Input: part model. Units: mm. Frame: model coordinates. A direction names the side the tool comes from. Round coordinates to 2 decimals unless told otherwise and drop trailing zeros. Loops run counter-clockwise (first coordinate to the right, second up) from the corner with the lowest first, then second, coordinate; pieces in that order, holes last.
1) First-contact query: pin 1 (1.9 mm diameter, centred on x = 11.5, y = -145, fed in from +Z) (3 decimals); pin 2 (1.9 mm diameter, centred on x = 12.5, z = -102.5, fed in from -Y); pin 3 (2.5 mm diameter, centred on x = 14, y = -114, fed in from -Z). Flat tips, straight axial feed; report the tip coordinate or a pass-through.
2) Access query for faces 1 (the face through (13, -114, -42.4)), 2 (the face through (13, -54, 0)), 3 (the face through (13, -146, -92.075)). Directions: +Z, -Z, +X, -X, +Y, -Y. A direction counts if a zero-diameter tool reaches every point of the face in a straight line with its end or side. Return the directions, or none.
3) Section D-D, the plane y = -138. Return loops of the section in (x, z), and give its area (3 significant figures).
4) Section C-C, the plane x = 13.5. State how many separate pieces and enclosed holes the cut face has, and give its area (3 significant figures).
5) Section A-A, the plane z = -25.4. Return loops of the section in (x, y), and give its area (3 significant figures).
6) Ray query, line 1 along Z through (x, y) = (12.5, -84); line 2 along Y through (x, z) = (11.75, -26); line 3 along Z through (x, y) = (10, -97.5). Return the intervals inside material, ascending.
7) Draft query along Y for faces 4 (the face through (13, -83, -42.4)), 5 (the face through (13, -140, 0)), 6 (the face through (13, -149.352, -86)), 7 (the face through (12.87, -118.09, -40.93)). Return one class per face: pulls with the +Y half, pulls with the -Y half, needs draft (parallel to the pull), parting line crosses it, or undercut.
8) Section B-B, the plane z = -9.9. Return loops of the section in (x, y).
from build123d import *

# Parameters (mm, degrees)
SKETCH1_W               = 44.958
SKETCH1_H               = 304.8
BOSS_EXTRUDE1_DEPTH     = 6.35
SKETCH2_W               = 6.35
SKETCH2_H               = 101.6
BOSS_EXTRUDE2_DEPTH     = 6.35
SKETCH3_W               = 120.65
SKETCH3_H               = 6.35
BOSS_EXTRUDE3_DEPTH     = 38.608
SKETCH8_W               = 6.35
SKETCH8_H               = 213.451350416
CUT_EXTRUDE4_DEPTH      = 1
CUT_EXTRUDE4_DEPTH_BACK = 134.35
SKETCH6_W               = 6.35
SKETCH6_H               = 12.7
CUT_EXTRUDE5_DEPTH      = 6.35
SKETCH4_3_W             = 6.35
SKETCH4_3_H             = 15.875
SKETCH4_3_H_2           = 6.35
CUT_EXTRUDE6_DEPTH      = 6.35


with BuildPart() as part:
    # Sketch1 → Boss-Extrude1 (new body)
    with BuildSketch(Plane.XY):
        with Locations((-6.477, 3.048)):
            Rectangle(SKETCH1_W, SKETCH1_H)
        with BuildLine():
            Line((-3.302, 133.858), (-3.302, -143.002))
            Line((-3.302, -143.002), (3.302, -143.002))
            Line((3.302, -143.002), (3.302, 143.002))
            Line((3.302, 143.002), (-16.256, 143.002))
            Line((-16.256, 143.002), (-16.256, 136.398))
            Line((-16.256, 136.398), (-5.842, 136.398))
            ThreePointArc((-5.842, 136.398), (-4.045948776, 135.654051224), (-3.302, 133.858))
        make_face(mode=Mode.SUBTRACT)
    extrude(amount=BOSS_EXTRUDE1_DEPTH)

    # Sketch2 → Boss-Extrude2 (add)
    with BuildSketch(Plane(origin=(16.002, 0, 0), x_dir=(0, 0, -1), z_dir=(1, 0, 0))):
        Polygon((120.65, -60.452), (120.65, -47.752), (0, -47.752), (0, -149.352), (120.65, -149.352), (120.65, -136.652), (127, -136.652), (127, -119.718666667), (120.65, -119.718666667), (120.65, -107.018666667), (127, -107.018666667), (127, -90.085333333), (120.65, -90.085333333), (120.65, -77.385333333), (127, -77.385333333), (127, -60.452), align=None)
        with BuildLine():
            ThreePointArc((11.4, -116.592), (9.9, -118.092), (8.4, -116.592))
            Line((8.4, -116.592), (8.4, -111.512))
            ThreePointArc((8.4, -111.512), (9.9, -110.012), (11.4, -111.512))
            Line((11.4, -111.512), (11.4, -116.592))
        make_face(mode=Mode.SUBTRACT)
        with BuildLine():
            Line((42.4, -111.512), (42.4, -116.592))
            ThreePointArc((42.4, -116.592), (40.9, -118.092), (39.4, -116.592))
            Line((39.4, -116.592), (39.4, -111.512))
            ThreePointArc((39.4, -111.512), (40.9, -110.012), (42.4, -111.512))
        make_face(mode=Mode.SUBTRACT)
        with BuildLine():
            ThreePointArc((36.4, -101.092), (25.4, -112.092), (14.4, -101.092))
            Line((14.4, -101.092), (14.4, -96.012))
            ThreePointArc((14.4, -96.012), (25.4, -85.012), (36.4, -96.012))
            Line((36.4, -96.012), (36.4, -101.092))
        make_face(mode=Mode.SUBTRACT)
        with BuildLine():
            ThreePointArc((11.4, -85.592), (9.9, -87.092), (8.4, -85.592))
            Line((8.4, -85.592), (8.4, -80.512))
            ThreePointArc((8.4, -80.512), (9.9, -79.012), (11.4, -80.512))
            Line((11.4, -80.512), (11.4, -85.592))
        make_face(mode=Mode.SUBTRACT)
        with BuildLine():
            ThreePointArc((42.4, -85.592), (40.9, -87.092), (39.4, -85.592))
            Line((39.4, -85.592), (39.4, -80.512))
            ThreePointArc((39.4, -80.512), (40.9, -79.012), (42.4, -80.512))
            Line((42.4, -80.512), (42.4, -85.592))
        make_face(mode=Mode.SUBTRACT)
        with Locations((-3.175, -98.552)):
            Rectangle(SKETCH2_W, SKETCH2_H)
    extrude(amount=-BOSS_EXTRUDE2_DEPTH)

    # Sketch3 → Boss-Extrude3 (add)
    with BuildSketch(Plane.ZY.offset(-9.652)):
        with Locations((-60.325, -146.177)):
            Rectangle(SKETCH3_W, SKETCH3_H)
    extrude(amount=BOSS_EXTRUDE3_DEPTH)

    # Sketch8 → Cut-Extrude4 (cut, two sides)
    with BuildSketch(Plane.XY.offset(6.35)) as cut_extrude4_sk:
        Polygon((-28.956, -149.352), (9.652, -149.352), (9.652, -47.752), (9.652, 155.448), (-28.956, 155.448), align=None)
        with BuildLine():
            Line((-16.256, 136.398), (-16.256, 143.002))
            Line((-16.256, 143.002), (3.302, 143.002))
            Line((3.302, 143.002), (3.302, -143.002))
            Line((3.302, -143.002), (-3.302, -143.002))
            Line((-3.302, -143.002), (-3.302, 133.858))
            ThreePointArc((-3.302, 133.858), (-4.045948776, 135.654051224), (-5.842, 136.398))
            Line((-5.842, 136.398), (-16.256, 136.398))
        make_face(mode=Mode.SUBTRACT)
        Polygon((-54.223542679, -149.352), (-28.956, -149.352), (-28.956, 155.448), (9.652, 155.448), (9.652, 165.699350416), (-54.223542679, 165.699350416), align=None)
        with Locations((12.827, 58.973675208)):
            Rectangle(SKETCH8_W, SKETCH8_H)
    extrude(amount=CUT_EXTRUDE4_DEPTH, mode=Mode.SUBTRACT)
    extrude(cut_extrude4_sk.sketch, amount=-CUT_EXTRUDE4_DEPTH_BACK, mode=Mode.SUBTRACT)

    # Sketch6 → Cut-Extrude5 (cut)
    with BuildSketch(Plane.XY.offset(6.35)):
        with Locations((12.827, -54.102)):
            Rectangle(SKETCH6_W, SKETCH6_H)
        with Locations((12.827, -83.735333333)):
            Rectangle(SKETCH6_W, SKETCH6_H)
        with Locations((12.827, -113.368666667)):
            Rectangle(SKETCH6_W, SKETCH6_H)
        with Locations((12.827, -143.002)):
            Rectangle(SKETCH6_W, SKETCH6_H)
    extrude(amount=-CUT_EXTRUDE5_DEPTH, mode=Mode.SUBTRACT)

    # Sketch4<3> → Cut-Extrude6 (cut)
    with BuildSketch(Plane.XZ.offset(149.352)):
        with Locations((12.827, -100.0125)):
            Rectangle(SKETCH4_3_W, SKETCH4_3_H)
        with Locations((12.827, -71.4375)):
            Rectangle(SKETCH4_3_W, SKETCH4_3_H)
        with Locations((12.827, -42.8625)):
            Rectangle(SKETCH4_3_W, SKETCH4_3_H)
        with Locations((12.827, -14.2875)):
            Rectangle(SKETCH4_3_W, SKETCH4_3_H)
        with Locations((12.827, 3.175)):
            Rectangle(SKETCH4_3_W, SKETCH4_3_H_2)
        with Locations((12.827, -3.175)):
            Rectangle(SKETCH4_3_W, SKETCH4_3_H_2)
    extrude(amount=-CUT_EXTRUDE6_DEPTH, mode=Mode.SUBTRACT)


solid = part.part
Final values:
1. pin 1: stops at z = -22.225
1. pin 2: stops at y = -143
1. pin 3: stops at z = -120.65
2. face 1: +X, -X
2. face 2: +Z, +X, -X, +Y
2. face 3: +X, -X, -Y
3. outline: (9.65, -120.65) - (16, -120.65) - (16, 0) - (9.65, 0) - close
3. area: 766 mm2
4. separate pieces: 1
4. enclosed holes: 5
4. area: 11,900 mm2
5. outline: (9.65, -149.35) - (16, -149.35) - (16, -112.09) - (9.65, -112.09) - close; (9.65, -85.01) - (16, -85.01) - (16, -47.75) - (9.65, -47.75) - close
5. area: 473 mm2
6. line 1: z = -120.65 to -42.4, -39.4 to -11.4, -8.4 to 0
6. line 2: y = -149.35 to -112.08, -85.03 to -47.75
6. line 3: z = -127 to -36.4, -14.4 to 6.35
7. face 4: undercut
7. face 5: needs draft
7. face 6: pulls with the -Y half
7. face 7: undercut
8. outline: (9.65, -143) - (16, -143) - (16, -118.09) - (9.65, -118.09) - close; (9.65, -110.01) - (16, -110.01) - (16, -87.09) - (9.65, -87.09) - close; (9.65, -79.01) - (16, -79.01) - (16, -47.75) - (9.65, -47.75) - close
